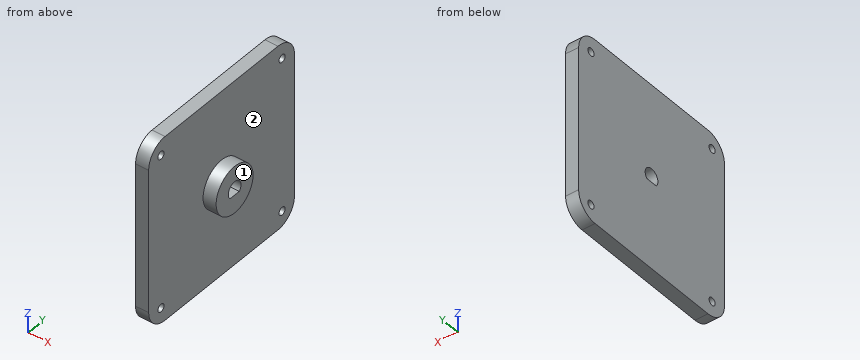
```python
from build123d import *

# Parameters (mm, degrees)
SKETCH1_W           = 71
SKETCH1_H           = 71
SKETCH1_R           = 1.5
BOSS_EXTRUDE1_DEPTH = 5
FILLET1_R           = 8
SKETCH2_R           = 9
BOSS_EXTRUDE2_DEPTH = 5
CUT_EXTRUDE1_DEPTH  = 11


with BuildPart() as part:
    # Sketch1 → Boss-Extrude1 (new body)
    with BuildSketch(Plane(origin=(0, 0, 0), x_dir=(0, 0, -1), z_dir=(1, 0, 0))):
        with Locations((35.5, 35.5)):
            Rectangle(SKETCH1_W, SKETCH1_H)
        with Locations((6, 6)):
            Circle(SKETCH1_R, mode=Mode.SUBTRACT)
        with Locations((6, 65)):
            Circle(SKETCH1_R, mode=Mode.SUBTRACT)
        with Locations((65, 65)):
            Circle(SKETCH1_R, mode=Mode.SUBTRACT)
        with Locations((65, 6)):
            Circle(SKETCH1_R, mode=Mode.SUBTRACT)
    extrude(amount=BOSS_EXTRUDE1_DEPTH)

    # Fillet1
    fillet1_edges = [part.edges().sort_by_distance(p)[0] for p in [
        (2.5, 71, 0),
        (2.5, 71, -71),
        (2.5, 0, -71),
        (2.5, 0, 0),
    ]]
    fillet(fillet1_edges, radius=FILLET1_R)

    # Sketch2 → Boss-Extrude2 (add)
    with BuildSketch(Plane(origin=(5, 0, 0), x_dir=(0, 0, -1), z_dir=(1, 0, 0))):
        with Locations((35.5, 35.5)):
            Circle(SKETCH2_R)
    extrude(amount=BOSS_EXTRUDE2_DEPTH)

    # Sketch3 → Cut-Extrude1 (cut, through all)
    with BuildSketch(Plane(origin=(10, 0, 0), x_dir=(0, 0, -1), z_dir=(1, 0, 0))):
        with BuildLine():
            Line((37.6, 33.21964915), (37.6, 37.78035085))
            ThreePointArc((37.6, 37.78035085), (32.4, 35.5), (37.6, 33.21964915))
        make_face()
    extrude(amount=-CUT_EXTRUDE1_DEPTH, mode=Mode.SUBTRACT)


solid = part.part
```
Work out the finished part from the listing and answer in its coordinate system (mm). Face numbers are marked on the shaded views. A direction names the side the tool comes from. Give positions to 0.01 mm unless a question says otherwise; leave off trailing zeros. Loops run counter-clockwise (first coordinate to the right, second up) from the corner with the lowest first, then second, coordinate; pieces in that order, holes last. Notation, with made-up numbers: M 16,36 L 42,36 A15 cw 42,54 Z; hole C 63.25,-30 d2. An arc over 180 degrees is marked long. One line per item, written item: value. Start each with the question number.
1. Find section A-A (z = -35.5). Give the vertices of the cut face in (x, y), and give its area (3 significant figures).
2. Each of these flat-tipped pins is pushed along its axis until it touches: P1, Ø3.5, axis at x = 7.5, y = 36, coming from the +Z side; P2, Ø5, axis at y = 6, z = -65, coming from the +X side. Where does it stop, or does it pass through?
3. Find the intervals of material crossed by probe 1 along Z at (x, y) = (3.1, 65); probe 2 along Y at (x, z) = (3, -7); probe 3 along Y at (x, z) = (4, -35.5), in increasing order.
4. Find section D-D (y = 6). Give the vertices of the cut face in (x, z), and give its area (3 significant figures).
5. Find section C-C (y = 35.5). Give the vertices of the cut face in (x, z).
6. Which of the six approach directions +Z, -Z, +X, -X, +Y, -Y give full straight-line access (tool end or side, diameter ignored) to the marked faces 1 and 2?
7. Find section B-B (x = 2.5). Give the vertices of the cut face in (y, z), and give its area (3 significant figures).
Reported:
1. outline: M 0,0 L 5,0 L 5,26.5 L 10,26.5 L 10,32.4 L 0,32.4 Z; M 0,38.6 L 10,38.6 L 10,44.5 L 5,44.5 L 5,71 L 0,71 Z
1. area: 383 mm²
2. P1: stops at z = -26.5
2. P2: stops at x = 5
3. probe 1: z = -70.75 to -66.5, -63.5 to -7.5, -4.5 to -0.25
3. probe 2: y = 0.06 to 4.88, 7.12 to 63.88, 66.12 to 70.94
3. probe 3: y = 0 to 32.4, 38.6 to 71
4. outline: M 0,-70.75 L 5,-70.75 L 5,-66.5 L 0,-66.5 Z; M 0,-63.5 L 5,-63.5 L 5,-7.5 L 0,-7.5 Z; M 0,-4.5 L 5,-4.5 L 5,-0.25 L 0,-0.25 Z
4. area: 322 mm²
5. outline: M 0,-71 L 5,-71 L 5,-44.5 L 10,-44.5 L 10,-37.6 L 0,-37.6 Z; M 0,-32.4 L 10,-32.4 L 10,-26.5 L 5,-26.5 L 5,0 L 0,0 Z
6. face 1: +Z, -Z, +X, +Y, -Y
6. face 2: +X
7. outline: M 0,-63 A8 ccw 8,-71 L 63,-71 A8 ccw 71,-63 L 71,-8 A8 ccw 63,0 L 8,0 A8 ccw 0,-8 Z; hole C 6,-65 d3; hole C 6,-6 d3; hole M 33.22,-37.6 L 37.78,-37.6 A3.1 ccw long Z; hole C 65,-65 d3; hole C 65,-6 d3
7. area: 4,930 mm²
